```python
from build123d import *

# Parameters (mm, degrees)
F1_DEPTH = 5
F2_R     = 2.49999
F3_W     = 5.486164242
F3_H     = 3.1326031312
F3_W_2   = 5.482269451
F3_W_3   = 2.8602015227
F3_H_2   = 9.1254087165
F3_H_3   = 2.179203555
F3_H_4   = 2.3905187845
F3_W_4   = 4.3584052473
F3_W_5   = 4.3584033847
F4_DEPTH = 25


# Not quite as in the source:
# - a fillet or chamfer is up to 0.001 mm smaller than in the source, because OpenCascade refuses the exact size


with BuildPart() as f1:
    # F0 (on Top) → F1 (new body)
    with BuildSketch(Plane.XY):
        with BuildLine():
            ThreePointArc((43.1041480843, -1.140358212), (41.4640780002, 0.7201286462), (40.168760519, 2.8351685639))
            Line((40.168760519, 2.8351685639), (-23.6701387912, 2.8351685639))
            Line((-23.6701387912, 2.8351685639), (-23.6701387912, 20.3415267169))
            Line((-23.6701387912, 20.3415267169), (-41.1761775613, 20.3415267169))
            Line((-41.1761775613, 20.3415267169), (-41.1761775613, 2.8351685639))
            Line((-41.1761775613, 2.8351685639), (-41.1761775613, -5.0545609556))
            Line((-41.1761775613, -5.0545609556), (40.2184031878, -5.0545609556))
            ThreePointArc((40.2184031878, -5.0545609556), (41.4937778577, -2.9739718927), (43.1041480843, -1.140358212))
        make_face()
        with BuildLine():
            ThreePointArc((67.3555774067, 8.7261943334), (67.3626426338, 8.9861285841), (67.3649979671, 9.246148169))
            ThreePointArc((67.3649979671, 9.246148169), (49.7178994981, 23.2169748342), (40.168760519, 2.8351685639))
            ThreePointArc((40.168760519, 2.8351685639), (41.4640780002, 0.7201286462), (43.1041480843, -1.140358212))
            ThreePointArc((43.1041480843, -1.140358212), (43.7292665999, -0.5749391558), (44.3865925628, -0.0473081805))
            ThreePointArc((44.3865925628, -0.0473081805), (47.9413125892, 20.8671965928), (65.6900889224, 9.2468057623))
            ThreePointArc((65.6900889224, 9.2468057623), (66.5335502723, 9.0207851567), (67.3555774067, 8.7261943334))
        make_face()
        with BuildLine():
            ThreePointArc((44.4356579567, -2.2642557619), (43.7528332621, -1.7225299618), (43.1041480843, -1.140358212))
            ThreePointArc((43.1041480843, -1.140358212), (41.4937778577, -2.9739718927), (40.2184031878, -5.0545609556))
            ThreePointArc((40.2184031878, -5.0545609556), (49.7174675435, -25.3901824255), (67.3204571559, -11.4652235061))
            ThreePointArc((67.3204571559, -11.4652235061), (67.3182526979, -11.2140597341), (67.3116400033, -10.96297335))
            ThreePointArc((67.3116400033, -10.96297335), (66.4614410979, -11.2621198468), (65.5889276735, -11.4880559652))
            ThreePointArc((65.5889276735, -11.4880559652), (47.9839421141, -22.9945229972), (44.4356579567, -2.2642557619))
        make_face()
        with BuildLine():
            ThreePointArc((73.9806472497, -1.1095376685), (72.169922865, 4.8199052741), (67.3555774067, 8.7261943334))
            ThreePointArc((67.3555774067, 8.7261943334), (67.3117311725, 8.010705268), (67.2322189831, 7.2982974448))
            ThreePointArc((67.2322189831, 7.2982974448), (71.1579723309, 3.8836422981), (72.6206968225, -1.1095376685))
            ThreePointArc((72.6206968225, -1.1095376685), (71.1453970138, -6.1222851765), (67.1899029185, -9.5366978003))
            ThreePointArc((67.1899029185, -9.5366978003), (67.2686178092, -10.2483123334), (67.3116400033, -10.96297335))
            ThreePointArc((67.3116400033, -10.96297335), (72.1566691186, -7.0586101253), (73.9806472497, -1.1095376685))
        make_face()
        with BuildLine():
            ThreePointArc((54.9590998914, -4.9748227507), (54.2466920753, -5.0543350042), (53.5312030139, -5.0981813027))
            ThreePointArc((53.5312030139, -5.0981813027), (58.3970374227, -10.4877579943), (65.5889276735, -11.4880559652))
            ThreePointArc((65.5889276735, -11.4880559652), (65.5889432165, -11.4766397403), (65.5889483975, -11.4652235061))
            ThreePointArc((65.5889483975, -11.4652235061), (65.5706384672, -10.7868000494), (65.5157619854, -10.1103518165))
            ThreePointArc((65.5157619854, -10.1103518165), (59.3188229712, -9.4308900821), (54.9590998914, -4.9748227507))
        make_face()
        with BuildLine():
            ThreePointArc((54.3661207024, 1.0392904692), (53.6782725799, 1.094777615), (52.9884165603, 1.1124562812))
            ThreePointArc((52.9884165603, 1.1124562812), (52.7533483797, -1.1613192361), (53.0105914352, -3.4326928652))
            ThreePointArc((53.0105914352, -3.4326928652), (53.7015001008, -3.4138898359), (54.3903575498, -3.3574650805))
            ThreePointArc((54.3903575498, -3.3574650805), (54.1133130855, -1.1605476943), (54.3661207024, 1.0392904692))
        make_face()
        with BuildLine():
            ThreePointArc((65.6900889395, 9.246148169), (65.6900889352, 9.2464769657), (65.6900889224, 9.2468057623))
            ThreePointArc((65.6900889224, 9.2468057623), (58.421880956, 8.2818061592), (53.5134993303, 2.8351685639))
            ThreePointArc((53.5134993303, 2.8351685639), (54.2281603431, 2.7921463054), (54.9397748692, 2.7134313507))
            ThreePointArc((54.9397748692, 2.7134313507), (59.3437953002, 7.2239168329), (65.6148612618, 7.867039641))
            ThreePointArc((65.6148612618, 7.867039641), (65.6712680509, 8.5555687863), (65.6900889395, 9.246148169))
        make_face()
        with BuildLine():
            ThreePointArc((60.2384014175, -1.1712057304), (60.9570485035, -0.6339967178), (61.6359032137, -0.0473081805))
            ThreePointArc((61.6359032137, -0.0473081805), (58.4654054664, 1.7637460297), (54.9397748692, 2.7134313507))
            ThreePointArc((54.9397748692, 2.7134313507), (54.6128353821, 1.8901056598), (54.3661207024, 1.0392904692))
            ThreePointArc((54.3661207024, 1.0392904692), (57.4423163149, 0.3061053356), (60.2384014175, -1.1712057304))
        make_face()
        with BuildLine():
            ThreePointArc((53.5134993303, 2.8351685639), (48.7018941946, 2.1796634707), (44.3865925628, -0.0473081805))
            ThreePointArc((44.3865925628, -0.0473081805), (45.0654472729, -0.6339967178), (45.7840943589, -1.1712057304))
            ThreePointArc((45.7840943589, -1.1712057304), (49.2106758058, 0.5245305343), (52.9884165603, 1.1124562812))
            ThreePointArc((52.9884165603, 1.1124562812), (53.2143527571, 1.9849696853), (53.5134993303, 2.8351685639))
        make_face()
        with BuildLine():
            ThreePointArc((44.3865925628, -0.0473081805), (43.7292665999, -0.5749391558), (43.1041480843, -1.140358212))
            ThreePointArc((43.1041480843, -1.140358212), (43.7528332621, -1.7225299618), (44.4356579567, -2.2642557619))
            ThreePointArc((44.4356579567, -2.2642557619), (45.0909975882, -1.6944412812), (45.7840943589, -1.1712057304))
            ThreePointArc((45.7840943589, -1.1712057304), (45.0654472729, -0.6339967178), (44.3865925628, -0.0473081805))
        make_face()
        with BuildLine():
            ThreePointArc((45.7840943589, -1.1712057304), (45.0909975882, -1.6944412812), (44.4356579567, -2.2642557619))
            ThreePointArc((44.4356579567, -2.2642557619), (48.7414590733, -4.4578309904), (53.5312030139, -5.0981813027))
            ThreePointArc((53.5312030139, -5.0981813027), (53.2366121166, -4.2761541948), (53.0105914352, -3.4326928652))
            ThreePointArc((53.0105914352, -3.4326928652), (49.2245751666, -2.854022082), (45.7840943589, -1.1712057304))
        make_face()
        with BuildLine():
            ThreePointArc((53.0105914352, -3.4326928652), (53.2366121166, -4.2761541948), (53.5312030139, -5.0981813027))
            ThreePointArc((53.5312030139, -5.0981813027), (54.2466920753, -5.0543350042), (54.9590998914, -4.9748227507))
            ThreePointArc((54.9590998914, -4.9748227507), (54.6371920778, -4.1793436416), (54.3903575498, -3.3574650805))
            ThreePointArc((54.3903575498, -3.3574650805), (53.7015001008, -3.4138898359), (53.0105914352, -3.4326928652))
        make_face()
        with BuildLine():
            ThreePointArc((54.9397748692, 2.7134313507), (54.2281603431, 2.7921463054), (53.5134993303, 2.8351685639))
            ThreePointArc((53.5134993303, 2.8351685639), (53.2143527571, 1.9849696853), (52.9884165603, 1.1124562812))
            ThreePointArc((52.9884165603, 1.1124562812), (53.6782725799, 1.094777615), (54.3661207024, 1.0392904692))
            ThreePointArc((54.3661207024, 1.0392904692), (54.6128353821, 1.8901056598), (54.9397748692, 2.7134313507))
        make_face()
        with BuildLine():
            ThreePointArc((54.9590998914, -4.9748227507), (58.4447091137, -4.0394696351), (61.5868378197, -2.2642557619))
            ThreePointArc((61.5868378197, -2.2642557619), (60.9314981882, -1.6944412812), (60.2384014175, -1.1712057304))
            ThreePointArc((60.2384014175, -1.1712057304), (57.4510535162, -2.6299259461), (54.3903575498, -3.3574650805))
            ThreePointArc((54.3903575498, -3.3574650805), (54.6371920778, -4.1793436416), (54.9590998914, -4.9748227507))
        make_face()
        with BuildLine():
            ThreePointArc((61.5868378197, -2.2642557619), (62.2696625143, -1.7225299618), (62.9183476921, -1.140358212))
            ThreePointArc((62.9183476921, -1.140358212), (62.2932291765, -0.5749391558), (61.6359032137, -0.0473081805))
            ThreePointArc((61.6359032137, -0.0473081805), (60.9570485035, -0.6339967178), (60.2384014175, -1.1712057304))
            ThreePointArc((60.2384014175, -1.1712057304), (60.9314981882, -1.6944412812), (61.5868378197, -2.2642557619))
        make_face()
        with BuildLine():
            ThreePointArc((62.9183476921, -1.140358212), (65.7918456304, 2.7126603808), (67.2322189831, 7.2982974448))
            ThreePointArc((67.2322189831, 7.2982974448), (66.4367398451, 7.6202051868), (65.6148612618, 7.867039641))
            ThreePointArc((65.6148612618, 7.867039641), (64.3390487935, 3.5510680946), (61.6359032137, -0.0473081805))
            ThreePointArc((61.6359032137, -0.0473081805), (62.2932291765, -0.5749391558), (62.9183476921, -1.140358212))
        make_face()
        with BuildLine():
            ThreePointArc((67.2322189831, 7.2982974448), (67.3117311725, 8.010705268), (67.3555774067, 8.7261943334))
            ThreePointArc((67.3555774067, 8.7261943334), (66.5335502723, 9.0207851567), (65.6900889224, 9.2468057623))
            ThreePointArc((65.6900889224, 9.2468057623), (65.6900889352, 9.2464769657), (65.6900889395, 9.246148169))
            ThreePointArc((65.6900889395, 9.246148169), (65.6712680509, 8.5555687863), (65.6148612618, 7.867039641))
            ThreePointArc((65.6148612618, 7.867039641), (66.4367398451, 7.6202051868), (67.2322189831, 7.2982974448))
        make_face()
        with BuildLine():
            ThreePointArc((67.1899029185, -9.5366978003), (65.7648954489, -4.9769306827), (62.9183476921, -1.140358212))
            ThreePointArc((62.9183476921, -1.140358212), (62.2696625143, -1.7225299618), (61.5868378197, -2.2642557619))
            ThreePointArc((61.5868378197, -2.2642557619), (64.2577141016, -5.8335676384), (65.5157619854, -10.1103518165))
            ThreePointArc((65.5157619854, -10.1103518165), (66.3665771981, -9.8636372133), (67.1899029185, -9.5366978003))
        make_face()
        with BuildLine():
            ThreePointArc((65.5889276735, -11.4880559652), (66.4614410979, -11.2621198468), (67.3116400033, -10.96297335))
            ThreePointArc((67.3116400033, -10.96297335), (67.2686178092, -10.2483123334), (67.1899029185, -9.5366978003))
            ThreePointArc((67.1899029185, -9.5366978003), (66.3665771981, -9.8636372133), (65.5157619854, -10.1103518165))
            ThreePointArc((65.5157619854, -10.1103518165), (65.5706384672, -10.7868000494), (65.5889483975, -11.4652235061))
            ThreePointArc((65.5889483975, -11.4652235061), (65.5889432165, -11.4766397403), (65.5889276735, -11.4880559652))
        make_face()
    extrude(amount=F1_DEPTH)

    # F2 (radius 2.5 in the source; OpenCascade refuses exactly that, so slightly less here)
    f2_edges = [f1.edges().sort_by_distance(p)[0] for p in [
        (-0.478887, -5.054561, 5),
        (-0.478887, -5.054561, 0),
        (8.249311, 2.835169, 5),
        (8.249311, 2.835169, 0),
    ]]
    fillet(f2_edges, radius=F2_R)

    # F3 (on face) → F4 (cut)
    with BuildSketch(Plane(origin=(0, 0, 0), x_dir=(1, 0, 0), z_dir=(0, 0, -1))):
        with Locations((-38.4330954403, -8.2126972266)):
            Rectangle(F3_W, F3_H)
        with Locations((-26.4112735167, -8.2126972266)):
            Rectangle(F3_W_2, F3_H)
        with Locations((-32.0807108656, -11.2091000192)):
            Rectangle(F3_W_3, F3_H_2)
        with Locations((-32.0807108656, -16.8614061549)):
            Rectangle(F3_W_3, F3_H_3)
        with Locations((-32.0807108656, -19.1462673247)):
            Rectangle(F3_W_3, F3_H_4)
        with Locations((-28.4714074805, -16.8614061549)):
            Rectangle(F3_W_4, F3_H_3)
        with Locations((-35.6900133193, -16.8614061549)):
            Rectangle(F3_W_5, F3_H_3)
    extrude(amount=-F4_DEPTH, mode=Mode.SUBTRACT)


solid = f1.part
```
Check sheet for the modelled part. Datum: model origin and axes. Units: mm. A direction names the side the tool comes from. Coordinates: 2 decimals unless noted, no trailing zeros. Loops run counter-clockwise (first coordinate to the right, second up) from the corner with the lowest first, then second, coordinate; pieces in that order, holes last. Notation, with made-up numbers: M 65,-16 L 94,-16 A23 ccw 94,1 Z; hole C 41.5,-14 d9. An arc over 180 degrees is marked long. Answer as a JSON object with one key per item and string values.
1. Sectioned sample at C-C on x = 59. Record the cut outline in (y, z).
Outcome:
{"outline": "M -24.46,0 L -22.53,0 L -22.53,5 L -24.46,5 Z; M -10.78,0 L -9.27,0 L -9.27,5 L -10.78,5 Z; M -3.8,0 L -1.93,0 L -1.93,5 L -3.8,5 Z; M -0.4,0 L 1.53,0 L 1.53,5 L -0.4,5 Z; M 7.05,0 L 8.56,0 L 8.56,5 L 7.05,5 Z; M 20.42,0 L 22.29,0 L 22.29,5 L 20.42,5 Z"}
2. Access from +Z, -Z, +X, -X, +Y, -Y to the whole of each face (thin tool, end or side, straight path). Record for faces 4 (the flat face through (-26, 6.646, 2)), 5 (the flat face through (-37, 20.342, 2)), 6 (the flat face through (-33.511, 11, 2)), 7 (the flat face through (-38, 6.646, 2)).
Outcome:
{"face 4": "+Z, -Z", "face 5": "+Z, -Z, -X, +Y", "face 6": "+Z, -Z, +Y", "face 7": "+Z, -Z, -X"}
3. Release check for a two-part mould opening along Y. For faces 1 (the flat face through (-27, 20.342, 2)), 2 (the flat face through (12, -1, 0)), 3 (the flat face through (-29, 17.951, 2)) record: pulls with the +Y half, pulls with the -Y half, needs draft (parallel to the pull), parting line crosses it, or undercut.
Outcome:
{"face 1": "pulls with the +Y half", "face 2": "needs draft", "face 3": "undercut"}
4. Depth check by flat-ended pin: P1, Ø1, axis at x = -23, y = 0.5, coming from the +Z side; P2, Ø1.5, axis at x = -35.5, z = 2.5, coming from the +Y side; P3, Ø1.3, axis at x = -35, z = 3.5, coming from the -Y side; P4, Ø1.5, axis at y = 17, z = 1.5, coming from the +X side. Enter the tip coordinate at first touch or a pass-through.
Outcome:
{"P1": "z = 5", "P2": "y = 20.34", "P3": "y = -5.03", "P4": "x = 65.54"}
5. Sectioned sample at B-B on y = -13. Record the cut outline in (x, z), and give its area (3 significant figures).
Outcome:
{"outline": "M 38.78,0 L 40.53,0 L 40.53,5 L 38.78,5 Z; M 65.49,0 L 67.24,0 L 67.24,5 L 65.49,5 Z", "area": "17.4 mm²"}
6. Scan lines: L1, parallel to X at y = 10, z = 0.5; L2, parallel to Y at x = 43, z = 1.45; L3, parallel to X at y = 4, z = 0.45. Record each from-to range of solid material in increasing order. Write a range as from..to.
Outcome:
{"L1": "-41.18..-33.51, -30.65..-23.67, 38.68..40.35, 65.67..67.35", "L2": "-21.69..-19.08, -3.85..1.47, 17.03..19.53", "L3": "-41.18..-23.67, 39.65..41.47, 54.06..55.65, 64.55..66.37, 71.08..72.67"}
